Verification items for this drawing (mm, ordinates from the low corner). A direction names the side the tool comes from. Round coordinates to 2 decimals unless told otherwise and drop trailing zeros. Write each loop counter-clockwise with the first axis right and the second up, starting at its lowest first coordinate (ties: lowest second). Pieces come first, ordered by that corner, then holes. Notation, with made-up numbers: (78, -14) -> (87, -14) arc R15 ccw to (87, 4) -> close; hole circle Ø8 at (77, 23.25). An arc over 180 degrees is marked (long way). Use one line per item in the form item = value. Start each with the question number.
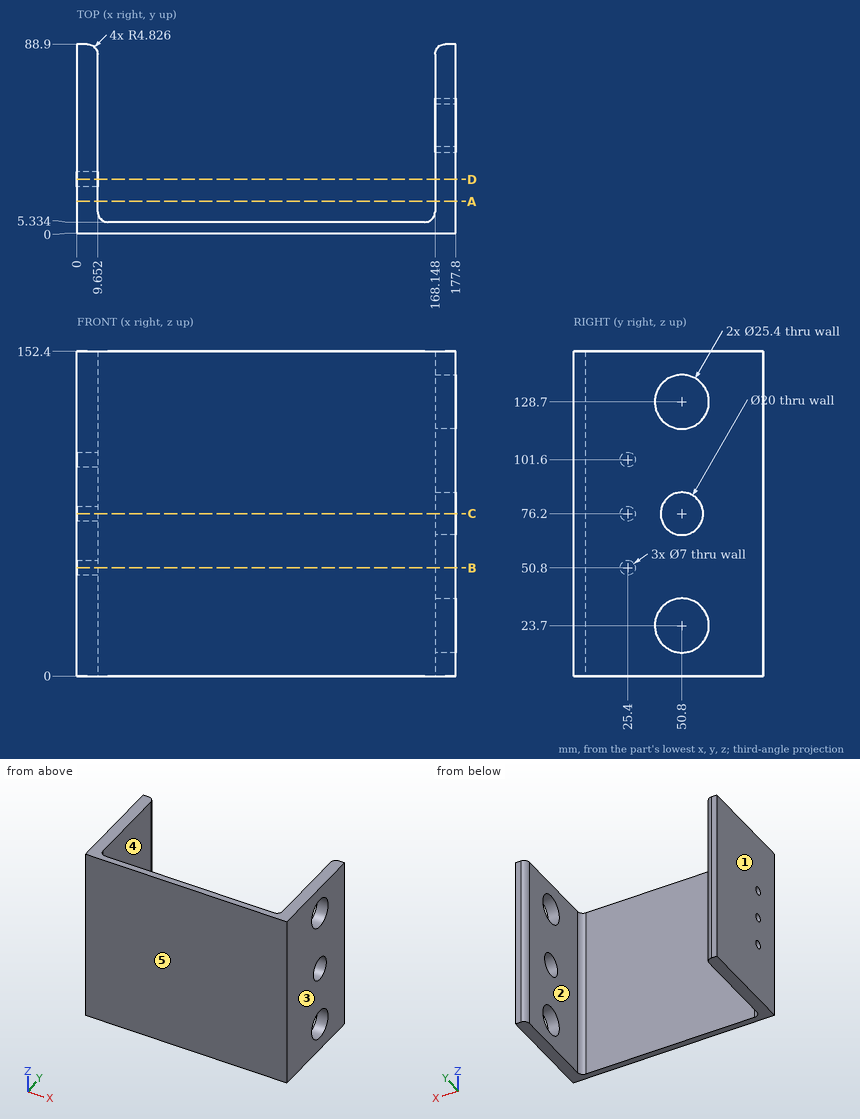
1. Tool access check on the marked faces 1 and 2. Record the directions out of +Z, -Z, +X, -X, +Y, -Y that give a thin tool (end or side, any length) a straight path to the whole face; none if there is none.
2. Scan lines: probe 1 along Z at (x, y) = (7, 25); probe 2 along Z at (x, y) = (171, 50); probe 3 along Y at (x, z) = (3.5, 50.8). Record each from-to range of solid material in increasing order.
3. Sectioned sample at C-C (z = 76.2). Enter the section's corners in (x, y), and give its area (3 significant figures).
4. Sectioned sample at B-B (z = 50.8). Enter the section's corners in (x, y).
5. Depth check by flat-ended pin: pin 1 (20.5 mm diameter, centred on y = 50.8, z = 23.7, fed in from -X); pin 2 (4 mm diameter, centred on x = 77, z = 61, fed in from +Y); pin 3 (6.5 mm diameter, centred on y = 25.4, z = 76.2, fed in from -X). Enter the tip coordinate at first touch or a pass-through.
6. Sectioned sample at D-D (y = 25.4). Enter the section's corners in (x, z), and give its area (3 significant figures).
7. Sectioned sample at A-A (y = 15). Enter the section's corners in (x, z), and give its area (3 significant figures).
8. Mould release check, pull along X, two halves, no side actions. Record for the marked faces 3, 4 and 5: +X half, -X half, draft (parallel to the pull), parting line (faces both ways), or undercut.
Returned:
q1.face_1 = +Z, -Z, -X, +Y, -Y
q1.face_2 = +Z, -Z, +Y
q2.probe_1 = 0 to 47.32, 54.28 to 72.72, 79.68 to 98.12, 105.08 to 152.4
q2.probe_2 = 0 to 11.03, 36.37 to 66.23, 86.17 to 116.03, 141.37 to 152.4
q2.probe_3 = 0 to 21.9, 28.9 to 88.9
q3.outline = (0, 0) -> (177.8, 0) -> (177.8, 40.8) -> (168.15, 40.8) -> (168.15, 10.16) arc R4.83 cw to (163.32, 5.33) -> (14.48, 5.33) arc R4.83 cw to (9.65, 10.16) -> (9.65, 21.9) -> (0, 21.9) -> close; (0, 28.9) -> (9.65, 28.9) -> (9.65, 84.07) arc R4.83 ccw to (4.83, 88.9) -> (0, 88.9) -> close; (168.15, 60.8) -> (177.8, 60.8) -> (177.8, 88.9) -> (172.97, 88.9) arc R4.83 ccw to (168.15, 84.07) -> close
q3.area = 2,300 mm^2
q4.outline = (0, 0) -> (177.8, 0) -> (177.8, 88.9) -> (172.97, 88.9) arc R4.83 ccw to (168.15, 84.07) -> (168.15, 10.16) arc R4.83 cw to (163.32, 5.33) -> (14.48, 5.33) arc R4.83 cw to (9.65, 10.16) -> (9.65, 21.9) -> (0, 21.9) -> close; (0, 28.9) -> (9.65, 28.9) -> (9.65, 84.07) arc R4.83 ccw to (4.83, 88.9) -> (0, 88.9) -> close
q5.pin_1 = 0
q5.pin_2 = 5.33
q5.pin_3 = 168.15
q6.outline = (0, 0) -> (9.65, 0) -> (9.65, 47.3) -> (0, 47.3) -> close; (0, 54.3) -> (9.65, 54.3) -> (9.65, 72.7) -> (0, 72.7) -> close; (0, 79.7) -> (9.65, 79.7) -> (9.65, 98.1) -> (0, 98.1) -> close; (0, 105.1) -> (9.65, 105.1) -> (9.65, 152.4) -> (0, 152.4) -> close; (168.15, 0) -> (177.8, 0) -> (177.8, 152.4) -> (168.15, 152.4) -> close
q6.area = 2,740 mm^2
q7.outline = (0, 0) -> (9.65, 0) -> (9.65, 152.4) -> (0, 152.4) -> close; (168.15, 0) -> (177.8, 0) -> (177.8, 152.4) -> (168.15, 152.4) -> close
q7.area = 2,940 mm^2
q8.face_3 = +X half
q8.face_4 = undercut
q8.face_5 = draft
